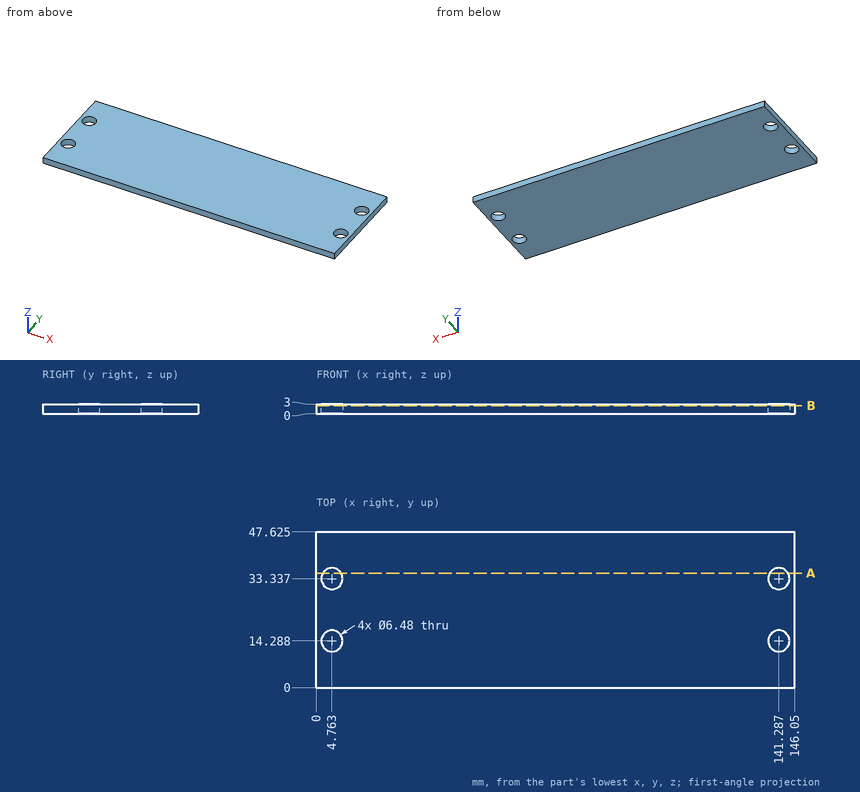
For this review, use the dimensioned drawing (mm, ordinates from the lowest corner) and the shaded views. Coordinates: 2 decimals unless noted, no trailing zeros. Loops run counter-clockwise (first coordinate to the right, second up) from the corner with the lowest first, then second, coordinate; pieces in that order, holes last. Notation, with made-up numbers: (83.25, -29) -> (131.25, -29) arc R33 cw to (131.25, 3) -> close; hole circle Ø8 at (28, -40). An arc over 180 degrees is marked (long way). Return JSON: item names as keys, results as strings. Group by question number.
(1) Consider section B-B, the plane z = 2.5. Give the boundary of the cut face in (x, y) (3 decimals), plus the area to 3 significant figures.
(2) Consider section A-A, the plane y = 35. Give the boundary of the cut face in (x, z), plus the area to 3 significant figures.
(3) To check wall thickness, follow L1, parallel to X at y = 33.5, z = 1.9; L2, parallel to X at y = 32, z = 1.65; L3, parallel to Y at x = 138.5, z = 1.1 (3 decimals). State the ranges of each line that lie inside material, in increasing order.
Results below:
{
 "1": {"outline": "(0, 0) -> (146.05, 0) -> (146.05, 47.625) -> (0, 47.625) -> close; hole circle Ø6.48 at (4.763, 14.288); hole circle Ø6.48 at (4.763, 33.337); hole circle Ø6.48 at (141.287, 14.288); hole circle Ø6.48 at (141.287, 33.337)", "area": "6,820 mm2"},
 "2": {"outline": "(0, 0) -> (1.98, 0) -> (1.98, 3) -> (0, 3) -> close; (7.54, 0) -> (138.51, 0) -> (138.51, 3) -> (7.54, 3) -> close; (144.07, 0) -> (146.05, 0) -> (146.05, 3) -> (144.07, 3) -> close", "area": "405 mm2"},
 "3": {"L1": "x = 0 to 1.53, 8 to 138.05, 144.52 to 146.05", "L2": "x = 0 to 1.81, 7.71 to 138.34, 144.24 to 146.05", "L3": "y = 0 to 12.636, 15.94 to 31.685, 34.989 to 47.625"}
}
